Design review of the part built by this model. Coordinates are the model's own, in mm. A direction names the side the tool comes from. Coordinates: 2 decimals unless noted, no trailing zeros. Write each loop counter-clockwise with the first axis right and the second up, starting at its lowest first coordinate (ties: lowest second). Pieces come first, ordered by that corner, then holes.
Q1. To check wall thickness, follow probe 1 along X at (y, z) = (7, 23.5); probe 2 along Y at (x, z) = (-4.5, 29); probe 3 along Z at (x, y) = (1.75, -8.5). State the ranges of each line that lie inside material, in increasing order.
Q2. Add section B-B, the plane x = -2.5. Give the boundary of the cut face in (y, z), plus the area to 4 significant figures.
Q3. Add section C-C, the plane z = 27. Give the boundary of the cut face in (x, y), plus the area to 4 significant figures.
Q4. The part is to be moulded in two halves that separate along Y. For faces 1 (the face through (0, 11.25, 22)), 2 (the face through (-5, 0, 23)), 3 (the face through (0, 0, 0)), say which applies: +Y half, -Y half, draft (parallel to the pull), parting line (faces both ways), or undercut.
Q5. Clearance check with a flat-ended pin moving along its axis: pin 1 Ø3 at (x, y) = (2.5, 0.5) entering from +Z. State where the tip first meets the part, or that it passes through.
Q6. Add section A-A, the plane y = 4. Give the boundary of the cut face in (x, z).
Q7. Machinability: for faces 4 (the face through (0, 0, 1.25)), 5 (the face through (-6.25, 0, 22)), which of the approach directions +Z, -Z, +X, -X, +Y, -Y give a long, thin tool a straight path to every point of the face, cutting with its end or side? Answer none if there is none.
Autodesk Inventor part; units mm, degrees
ref_plane "YZ Plane" through (0, 0, 0) normal (1, 0, 0) x (0, 1, 0)
ref_plane "XZ Plane" through (0, 0, 0) normal (0, 1, 0) x (-1, 0, 0)
ref_plane "XY Plane" through (0, 0, 0) normal (0, 0, 1) x (1, 0, 0)
sketch "Sketch1" plane through (0, 0, 0) normal (0, 0, 1) x (1, 0, 0)
  line L0 (0, 15.75) -> (0, -15.75) construction
  line L1 (-8.75, 0) -> (8.75, 0) construction
  line L2 (-6.25, 11.25) -> (6.25, 11.25)
  line L3 (6.25, 11.25) -> (6.25, -11.25)
  line L4 (6.25, -11.25) -> (-6.25, -11.25)
  line L5 (-6.25, -11.25) -> (-6.25, 11.25)
  point P0 (0, 0)
  dimension "d0" = 22.5
  dimension "d1" = 12.5
extrude "Extrusion1" add sketch "Sketch1" along normal blind 45
sketch "Sketch2" plane through (0, 0, 45) normal (0, 0, 1) x (1, 0, 0)
  line L0 (-6.25, 11.25) -> (6.25, 11.25)
  line L1 (-6.25, -11.25) -> (-6.25, 11.25)
  line L2 (-5, 10) -> (5, 10)
  line L3 (5, 10) -> (5, -10)
  line L4 (5, -10) -> (-5, -10)
  line L5 (-5, -10) -> (-5, 10)
  point P0 (0, 0)
  dimension "d4" = 10
  dimension "d5" = 20
  dimension "d6" = 1.25
  dimension "d7" = 1.25
extrude "Extrusion2" cut sketch "Sketch2" against normal blind 43.75
properties part number "Küvette_20mm" material "Glass"
Here are the results:
1. probe 1: x = -6.25 to -5, 5 to 6.25
1. probe 2: y = -11.25 to -10, 10 to 11.25
1. probe 3: z = 0 to 1.25
2. outline: (-11.25, 0) - (11.25, 0) - (11.25, 45) - (10, 45) - (10, 1.25) - (-10, 1.25) - (-10, 45) - (-11.25, 45) - close
2. area: 137.5 mm2
3. outline: (-6.25, -11.25) - (6.25, -11.25) - (6.25, 11.25) - (-6.25, 11.25) - close; hole (-5, -10) - (5, -10) - (5, 10) - (-5, 10) - close
3. area: 81.25 mm2
4. face 1: +Y half
4. face 2: undercut
4. face 3: draft
5. pin 1: stops at z = 1.25
6. outline: (-6.25, 0) - (6.25, 0) - (6.25, 45) - (5, 45) - (5, 1.25) - (-5, 1.25) - (-5, 45) - (-6.25, 45) - close
7. face 4: +Z
7. face 5: +Z, -Z, -X, +Y, -Y
